```python
from build123d import *

# Parameters (mm, degrees)
SKETCH1_R           = 44.45
BOSS_EXTRUDE1_DEPTH = 57.15
BOSS_EXTRUDE2_DEPTH = 25.4


with BuildPart() as part:
    # Sketch1 → Boss-Extrude1 (new body)
    with BuildSketch(Plane(origin=(0, 0, 0), x_dir=(1, 0, 0), z_dir=(0, 1, 0))):
        Circle(SKETCH1_R)
    extrude(amount=BOSS_EXTRUDE1_DEPTH)

    # Sketch3 → Boss-Extrude2 (add)
    with BuildSketch(Plane(origin=(0, 6.35, 0), x_dir=(1, 0, 0), z_dir=(0, 1, 0))):
        with BuildLine():
            ThreePointArc((25.93836289, 36.097144355), (41.652954947, 15.518822255), (43.234152204, -10.325240105))
            add(Edge.make_bspline(
                [(107.47145922, -21.303368675), (79.942418966, 7.909262822), (43.234152204, -10.325240105)],
                knots=[0, 0, 0, 1, 1, 1], degree=2))
            add(Edge.make_bspline(
                [(25.93836289, 36.097144355), (62.849269779, 44.250068413), (102.789157255, 15.374374685), (107.47145922, -21.303368675)],
                knots=[0, 0, 0, 0, 1, 1, 1, 1], degree=3))
        make_face()
        with BuildLine():
            ThreePointArc((-25.93836289, -36.097144355), (-41.652954947, -15.518822255), (-43.234152204, 10.325240105))
            add(Edge.make_bspline(
                [(-107.47145922, 21.303368675), (-79.942418966, -7.909262822), (-43.234152204, 10.325240105)],
                knots=[0, 0, 0, 1, 1, 1], degree=2))
            add(Edge.make_bspline(
                [(-25.93836289, -36.097144355), (-62.849269779, -44.250068413), (-102.789157255, -15.374374685), (-107.47145922, 21.303368675)],
                knots=[0, 0, 0, 0, 1, 1, 1, 1], degree=3))
        make_face()
    extrude(amount=BOSS_EXTRUDE2_DEPTH)


solid = part.part
```
Part model, mm, in its own coordinate system. Coordinates: 2 decimals unless noted, no trailing zeros. Order: outer loops, then holes, each group sorted by start corner. A loop starts at its lowest first (then second) coordinate and runs counter-clockwise, first axis right, second up. Notation, with made-up numbers: (8.25, 72) - (67.25, 72) arc R27 ccw to (67.25, 111) - close; hole circle Ø10 at (28, 19.25). An arc over 180 degrees is marked (long way). Return JSON: item names as keys, results as strings. Group by question number.
Item 1: Pin check, flat tips, straight feed: pin 1 (4 mm diameter, centred on x = 64.5, y = 17.5, fed in from -Z); pin 2 (8 mm diameter, centred on y = 12, z = -33, fed in from +X); pin 3 (1.5 mm diameter, centred on x = -37.5, y = 50, fed in from -Z); pin 4 (3 mm diameter, centred on x = 26, z = 3.5, fed in from -Y). Stop position of each tip, or through.
Item 2: Cut at A-A (y = 35.5). List the corners of the cut face in (x, z).
Item 3: Drill centre lines: probe 1 along Y at (x, z) = (98.5, 13); probe 2 along X at (y, z) = (15.5, -14); probe 3 along Z at (x, y) = (-10.5, 24). Where is each one in solid material? Low to high. Write a range as from..to.
Item 4: Cut at B-B (x = -9). List the corners of the cut face in (y, z), plus the area to 3 significant figures.
Check values:
{
 "1": {"pin 1": "stops at z = -32.97", "pin 2": "stops at x = 71.1", "pin 3": "stops at z = -25", "pin 4": "stops at y = 0"},
 "2": {"outline": "circle Ø88.9 at (0, 0)"},
 "3": {"probe 1": "y = 6.35..31.75", "probe 2": "x = -106.06..-99.51, -42.19..90.41", "probe 3": "z = -43.19..43.19"},
 "4": {"outline": "(0, -43.53) - (57.15, -43.53) - (57.15, 43.53) - (0, 43.53) - close", "area": "4,980 mm2"}
}
